```python
from build123d import *

# Parameters (mm, degrees)
ESQUISSE1_W             = 8
ESQUISSE1_H             = 7
BOSS_EXTRU_1_DEPTH      = 1
ESQUISSE2_W             = 1
ESQUISSE2_H             = 7
BOSS_EXTRU_2_DEPTH      = 9
ESQUISSE3_R             = 1.5
ENL_V_MAT_EXTRU_1_DEPTH = 14.304134696
ESQUISSE4_R             = 1.5
ENL_V_MAT_EXTRU_2_DEPTH = 12.747340124


with BuildPart() as part:
    # Esquisse1 → Boss.-Extru.1 (new body)
    with BuildSketch(Plane.XY):
        with Locations((0, 3.5)):
            Rectangle(ESQUISSE1_W, ESQUISSE1_H)
    extrude(amount=BOSS_EXTRU_1_DEPTH)

    # Esquisse2 → Boss.-Extru.2 (add)
    with BuildSketch(Plane.XY.offset(1)):
        with Locations((-4.5, 3.5)):
            Rectangle(ESQUISSE2_W, ESQUISSE2_H)
    extrude(amount=-BOSS_EXTRU_2_DEPTH)

    # Esquisse3 → Enlèv. mat.-Extru.1 (cut, through all)
    with BuildSketch(Plane(origin=(-4, 0, 0), x_dir=(0, 0, -1), z_dir=(1, 0, 0))):
        with Locations(Location((4, 3.5, 0), (0, 0, 90))):
            Circle(ESQUISSE3_R)
    extrude(amount=-ENL_V_MAT_EXTRU_1_DEPTH, mode=Mode.SUBTRACT)

    # Esquisse4 → Enlèv. mat.-Extru.2 (cut, through all)
    with BuildSketch(Plane(origin=(0, 0, 0), x_dir=(-1, 0, 0), z_dir=(0, 0, -1))):
        with Locations((0, 3.5)):
            Circle(ESQUISSE4_R)
    extrude(amount=-ENL_V_MAT_EXTRU_2_DEPTH, mode=Mode.SUBTRACT)


solid = part.part
```
Part model, mm, in its own coordinate system. A direction names the side the tool comes from. Round coordinates to 2 decimals unless told otherwise and drop trailing zeros. Write each loop counter-clockwise with the first axis right and the second up, starting at its lowest first coordinate (ties: lowest second). Pieces come first, ordered by that corner, then holes. Notation, with made-up numbers: (-10, -24) -> (5, -24) arc R23 cw to (5, -10) -> close; hole circle Ø9 at (17.5, 25.25). An arc over 180 degrees is marked (long way). Return JSON: item names as keys, results as strings. Group by question number.
Q1. Saw through at C-C on y = 3.5. Write the cut outline in (x, z).
Q2. Mould opens along X. For faces 3 (the flat face through (-4.2, 7, -1.5)), 4 (the cylindrical face through (1.5, 3.57, 0.49)), 5 (the flat face through (4, 3.5, 0.5)) say: pulls with the +X half, pulls with the -X half, needs draft (parallel to the pull), parting line crosses it, or undercut.
Q3. Probe L1, parallel to Z at x = -4.55, y = 3.5; L2, parallel to Y at x = 0, z = 0.45; L3, parallel to Z at x = -2.25, y = 4.5. List the from-to ranges inside material, lowest first. Write a range as [from, to].
Q4. Pin check, flat tip, straight feed: pin 1 (3 mm diameter, centred on x = -2, y = 1.5, fed in from -Z). Stop position of the tip, or through.
Q5. Saw through at A-A on x = 0. Write the cut outline in (y, z).
Q6. Which spindle directions (+Z, -Z, +X, -X, +Y, -Y) get a long thin tool onto all of the face, cutting with end or side? Do faces 1 (the flat face through (-2, 4, 0)), 2 (the flat face through (-4.5, 3.5, -8)). Say none if no direction does.
Q7. Saw through at B-B on z = -4. Write the cut outline in (x, y), plus the area to 3 significant figures.
Q8. Saw through at D-D on y = 1.5. Write the cut outline in (x, z).
Answer:
{
 "1": {"outline": "(-5, -8) -> (-4, -8) -> (-4, -5.5) -> (-5, -5.5) -> close; (-5, -2.5) -> (-4, -2.5) -> (-4, 0) -> (-1.5, 0) -> (-1.5, 1) -> (-5, 1) -> close; (1.5, 0) -> (4, 0) -> (4, 1) -> (1.5, 1) -> close"},
 "2": {"face 3": "needs draft", "face 4": "undercut", "face 5": "pulls with the +X half"},
 "3": {"L1": "[-8, -5.5], [-2.5, 1]", "L2": "[0, 2], [5, 7]", "L3": "[0, 1]"},
 "4": {"pin 1": "z = 0"},
 "5": {"outline": "(0, 0) -> (2, 0) -> (2, 1) -> (0, 1) -> close; (5, 0) -> (7, 0) -> (7, 1) -> (5, 1) -> close"},
 "6": {"face 1": "-Z, +X, +Y, -Y", "face 2": "-Z, +X, -X, +Y, -Y"},
 "7": {"outline": "(-5, 0) -> (-4, 0) -> (-4, 2) -> (-5, 2) -> close; (-5, 5) -> (-4, 5) -> (-4, 7) -> (-5, 7) -> close", "area": "4.00 mm2"},
 "8": {"outline": "(-5, -8) -> (-4, -8) -> (-4, 0) -> (4, 0) -> (4, 1) -> (-5, 1) -> close"}
}
